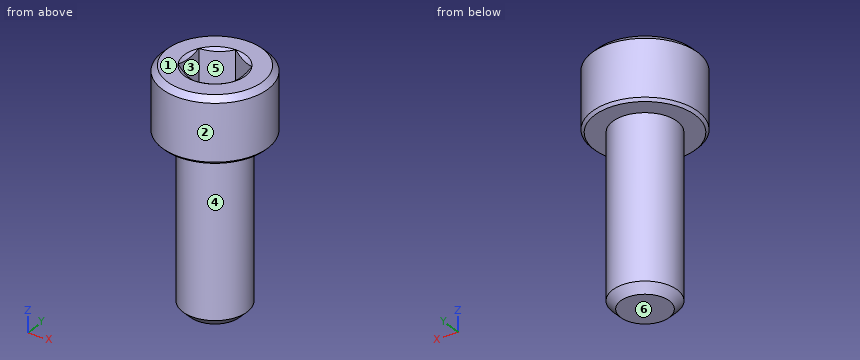
```python
from build123d import *

# Parameters (mm, degrees)
CUT_EXTRUDE1_DEPTH = 2.9765625
CHAMFER1_SIZE      = 0.396875
CHAMFER2_SIZE      = 0.1984375


with BuildPart() as part:
    # Sketch2 → Revolve1 (revolve)
    with BuildSketch(Plane(origin=(0, 0, 0), x_dir=(0, 0, -1), z_dir=(1, 0, 0)), mode=Mode.PRIVATE) as revolve1_sk:
        Polygon((8.763, 1.8176875), (8.1676875, 2.413), (-3.937, 2.413), (-3.937, 3.96875), (-8.763, 3.96875), (-8.763, 0), (8.763, 0), align=None)
    revolve(revolve1_sk.sketch.rotate(Axis((0, 0, -8.763), (0, 0, 1)), 90), axis=Axis((0, 0, -8.763), (0, 0, 1)))

    # Sketch4 → Cut-Extrude1 (cut)
    with BuildSketch(Plane.XY.offset(8.763)):
        Polygon((0, 2.291358881), (-1.984375, 1.14567944), (-1.984375, -1.14567944), (0, -2.291358881), (1.984375, -1.14567944), (1.984375, 1.14567944), align=None)
    extrude(amount=-CUT_EXTRUDE1_DEPTH, mode=Mode.SUBTRACT)

    # Cut-Extrude2 cone 1 section (on through the dimple's axis) → Cut-Extrude2 (revolve, cut)
    with BuildSketch(Plane(origin=(0, 0, 8.763), x_dir=(0, -1, 0), z_dir=(1, 0, 0))):
        Polygon((0, 0), (2.291358881, 0), (0, 1.322916667), align=None)
    revolve(axis=Axis((0, 0, 8.763), (0, 0, -1)), mode=Mode.SUBTRACT)

    # Chamfer1
    chamfer1_edges = [part.edges().sort_by_distance(p)[0] for p in [
        (3.96875, 0, 8.763),
    ]]
    chamfer(chamfer1_edges, length=CHAMFER1_SIZE)

    # Chamfer2
    chamfer2_edges = [part.edges().sort_by_distance(p)[0] for p in [
        (3.96875, 0, 3.937),
    ]]
    chamfer(chamfer2_edges, length=CHAMFER2_SIZE)


solid = part.part
```
Part model, mm, in its own coordinate system. Face numbers are marked on the shaded views. A direction names the side the tool comes from. Round coordinates to 2 decimals unless told otherwise and drop trailing zeros. Loops run counter-clockwise (first coordinate to the right, second up) from the corner with the lowest first, then second, coordinate; pieces in that order, holes last.
Item 1: Cut at B-B, the plane z = -4.5. Give the cut face in (x, y), then the cut area to 3 significant figures.
Item 2: Cut at A-A, the plane y = 0. Give the cut face in (x, z).
Item 3: 3-axis set-ups, long thin cutter, end or side, ignore diameter. For the marked faces 4, 5 and 6: which of +Z, -Z, +X, -X, +Y, -Y reach the whole face in a straight line?
Item 4: Drop flat-ended pins along their axis: P1, Ø4, axis at y = 2.5, z = -5.5, coming from the +X side; P2, Ø2, axis at x = -2, z = 6.5, coming from the -Y side; P3, Ø0.7, axis at y = 0.5, z = 7, coming from the +X side. Give the stop position or say it passes through.
Item 5: Mould opens along Y. For the marked faces 1, 2 and 3 say: +Y half, -Y half, draft (parallel to the pull), parting line (faces both ways), or undercut.
Item 6: Drill centre lines: line 1 (X direction, y = 0.75, z = -4.75); line 2 (X direction, y = -0.5, z = 8.25); line 3 (Z direction, x = -3, y = 1.5). Where is each one in solid material? Low to high.
A:
1. outline: circle Ø4.83 at (0, 0)
1. area: 18.3 mm2
2. outline: (-3.97, 4.14) - (-3.77, 3.94) - (-2.41, 3.94) - (-2.41, -8.17) - (-1.82, -8.76) - (1.82, -8.76) - (2.41, -8.17) - (2.41, 3.94) - (3.77, 3.94) - (3.97, 4.14) - (3.97, 8.37) - (3.57, 8.76) - (2.29, 8.76) - (1.98, 8.59) - (1.98, 5.79) - (-1.98, 5.79) - (-1.98, 8.59) - (-2.29, 8.76) - (-3.57, 8.76) - (-3.97, 8.37) - close
3. face 4: -Z
3. face 5: +Z
3. face 6: -Z, +X, -X, +Y, -Y
4. P1: stops at x = 2.36
4. P2: stops at y = -3.84
4. P3: stops at x = 3.97
5. face 1: draft
5. face 2: parting line
5. face 3: undercut
6. line 1: x = -2.29 to 2.29
6. line 2: x = -3.94 to -1.98, 1.98 to 3.94
6. line 3: z = 3.94 to 8.76
